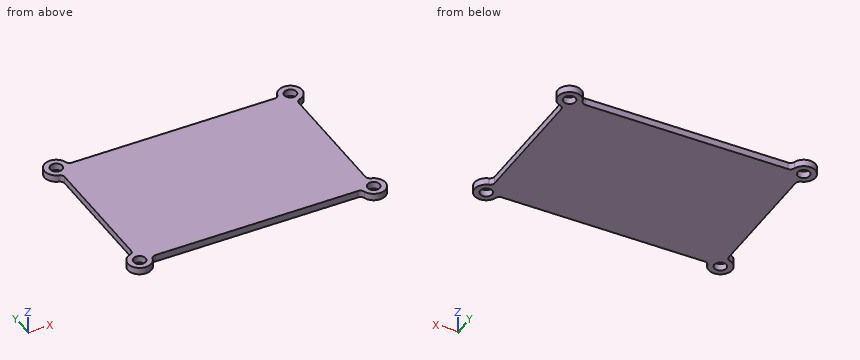
from build123d import *

# Parameters (mm, degrees)
SKETCH_1_R      = 1.55
EXTRUDE_1_DEPTH = 1.8


with BuildPart() as part:
    # 草图1 → 凸台-拉伸1 (new body)
    with BuildSketch(Plane.XY):
        with BuildLine():
            ThreePointArc((0, 35.937980798), (-0.244500417, 36.680591455), (-0.882352941, 37.132692328))
            ThreePointArc((-0.882352941, 37.132692328), (-2.121320344, 42.121320344), (2.867307672, 40.882352941))
            ThreePointArc((2.867307672, 40.882352941), (3.319408545, 40.244500417), (4.062019202, 40))
            Line((4.062019202, 40), (55.937980798, 40))
            ThreePointArc((55.937980798, 40), (56.680591455, 40.244500417), (57.132692328, 40.882352941))
            ThreePointArc((57.132692328, 40.882352941), (62.121320344, 42.121320344), (60.882352941, 37.132692328))
            ThreePointArc((60.882352941, 37.132692328), (60.244500417, 36.680591455), (60, 35.937980798))
            Line((60, 35.937980798), (60, 4.062019202))
            ThreePointArc((60, 4.062019202), (60.244500417, 3.319408545), (60.882352941, 2.867307672))
            ThreePointArc((60.882352941, 2.867307672), (62.121320344, -2.121320344), (57.132692328, -0.882352941))
            ThreePointArc((57.132692328, -0.882352941), (56.680591455, -0.244500417), (55.937980798, 0))
            Line((55.937980798, 0), (4.062019202, 0))
            ThreePointArc((4.062019202, 0), (3.319408545, -0.244500417), (2.867307672, -0.882352941))
            ThreePointArc((2.867307672, -0.882352941), (-2.121320344, -2.121320344), (-0.882352941, 2.867307672))
            ThreePointArc((-0.882352941, 2.867307672), (-0.244500417, 3.319408545), (0, 4.062019202))
            Line((0, 4.062019202), (0, 35.937980798))
        make_face()
        Circle(SKETCH_1_R, mode=Mode.SUBTRACT)
        with Locations((60, 0)):
            Circle(SKETCH_1_R, mode=Mode.SUBTRACT)
        with Locations((60, 40)):
            Circle(SKETCH_1_R, mode=Mode.SUBTRACT)
        with Locations((0, 40)):
            Circle(SKETCH_1_R, mode=Mode.SUBTRACT)
    extrude(amount=EXTRUDE_1_DEPTH)


solid = part.part
Work out the finished part from the listing and answer in its coordinate system (mm). Round coordinates to 2 decimals unless told otherwise and drop trailing zeros. Write each loop counter-clockwise with the first axis right and the second up, starting at its lowest first coordinate (ties: lowest second). Pieces come first, ordered by that corner, then holes. Notation, with made-up numbers: (89.5, -39) -> (100.5, -39) arc R15 ccw to (100.5, -28) -> close; hole circle Ø9 at (85.25, 9). An arc over 180 degrees is marked (long way). Answer as CSV lines item,"result". Start each with the question number.
(1) The part is cut by section B-B, the plane y = 17. Give the vertices of the cut face in (x, z).
(2) The part is cut by section A-A, the plane z = 0.45. Give the vertices of the cut face in (x, y), then the cut area to 3 significant figures.
(3) Each of these flat-tipped pins is pushed along its axis until it touches: pin 1 (0.9 mm diameter, centred on x = 40, z = 1.5, fed in from -Y); pin 2 (0.9 mm diameter, centred on y = 23, z = 1.5, fed in from +X); pin 3 (0.9 mm diameter, centred on x = 30.5, z = 1, fed in from +Y). Where does it stop, or does it pass through?
(4) The part is cut by section C-C, the plane x = 16.5. Give the vertices of the cut face in (y, z).
(5) Find the intervals of material crossed by probe 1 along Y at (x, z) = (51, 0.6); probe 2 along X at (y, z) = (23, 1.75), in increasing order.
Output values:
1,outline,"(0, 0) -> (60, 0) -> (60, 1.8) -> (0, 1.8) -> close"
2,outline,"(-0.88, 2.87) arc R3 ccw (long way) to (2.87, -0.88) arc R1.25 cw to (4.06, 0) -> (55.94, 0) arc R1.25 cw to (57.13, -0.88) arc R3 ccw (long way) to (60.88, 2.87) arc R1.25 cw to (60, 4.06) -> (60, 35.94) arc R1.25 cw to (60.88, 37.13) arc R3 ccw (long way) to (57.13, 40.88) arc R1.25 cw to (55.94, 40) -> (4.06, 40) arc R1.25 cw to (2.87, 40.88) arc R3 ccw (long way) to (-0.88, 37.13) arc R1.25 cw to (0, 35.94) -> (0, 4.06) arc R1.25 cw to start; hole circle Ø3.1 at (0, 0); hole circle Ø3.1 at (0, 40); hole circle Ø3.1 at (60, 0); hole circle Ø3.1 at (60, 40)"
2,area,"2,460 mm²"
3,pin 1,"stops at y = 0"
3,pin 2,"stops at x = 60"
3,pin 3,"stops at y = 40"
4,outline,"(0, 0) -> (40, 0) -> (40, 1.8) -> (0, 1.8) -> close"
5,probe 1,"y = 0 to 40"
5,probe 2,"x = 0 to 60"
